Autodesk Inventor part; units mm, degrees
ref_plane "YZ Plane" through (0, 0, 0) normal (1, 0, 0) x (0, 1, 0)
ref_plane "XZ Plane" through (0, 0, 0) normal (0, 1, 0) x (-1, 0, 0)
ref_plane "XY Plane" through (0, 0, 0) normal (0, 0, 1) x (1, 0, 0)
sketch "Sketch1" plane through (0, 0, 0) normal (0, 0, 1) x (1, 0, 0)
  circle A0 centre (0, 0) radius 25
  circle A1 centre (0, 0) radius 23
  circle A2 centre (0, 0) radius 22
  circle A3 centre (0, 0) radius 20
  circle A4 centre (0, 0) radius 19
  circle A5 centre (0, 0) radius 17
  line L0 (25, 0) -> (-25, 0) construction
  line L1 (0, 25) -> (0, -25) construction
  dimension "d0" = 50
  dimension "d1" = 2
  dimension "d2" = 44
  dimension "d3" = 2
  dimension "d4" = 38
  dimension "d5" = 2
extrude "Extrusion2" add sketch "Sketch1" along normal blind 10 contours A0
sketch "Sketch2" plane through (0, 0, 0) normal (0, 1, 0) x (-1, 0, 0)
  line L0 (-23, 0) -> (23, 0) construction
  line L1 (23, 0) -> (-23, 0) construction
  line L2 (-23, 0) -> (-23, 10) construction
  line L3 (23, 10) -> (23, 0) construction
  line L4 (23, 10) -> (23, 0) construction
  circle A0 centre (23, 5) radius 2 construction
  line L5 (0, 0) -> (0, 10) construction
  circle A1 centre (-23, 5) radius 2 construction
  line L6 (24.0412, 3.2924) -> (23, 7)
  line L7 (-23, 0) -> (-23, 10)
  line L8 (23, 10) -> (23, 0) construction
  line L9 (-23, 5) -> (23, 5) construction
  line L10 (23, 10) -> (23, 0) construction
  circle A2 centre (-22.1677, 5) radius 2
  circle A3 centre (22.2113, 5) radius 2
  line L11 (20.2113, 5) -> (24.2113, 5)
  line L12 (-20.1677, 5) -> (-24.1677, 5)
  point P0 (-23, 7)
  point P1 (-23, 3)
  dimension "d12" = 4
  dimension "d11" = 10
  dimension "d31" = 46
  dimension "d32" = 4
  dimension "d33" = 4
revolve "Revolution1" add sketch "Sketch2" angle 360 about axis through (23, 0, 5) along (-1, 0, 0) picked at (21.3446, 5.1473) picked at (23.3511, 6.1311) contours L11 A3 L6 | L6 A3 L11
revolve "Revolution2" add sketch "Sketch2" angle 360 about axis through (23, 0, 5) along (-1, 0, 0) picked at (-23.13, 6.1339) picked at (-21.1282, 5.1469) contours L12 A2 L7 | L7 A2 L12
properties part number "probe_gimbal_prototype"
CAD build for the part. Positions are in the model's coordinates, mm. Coordinates: 2 decimals unless noted, no trailing zeros. Write each loop counter-clockwise with the first axis right and the second up, starting at its lowest first coordinate (ties: lowest second). Pieces come first, ordered by that corner, then holes. Notation, with made-up numbers: (7.25, 71.25) -> (28.25, 71.25) arc R11 ccw to (28.25, 84.25) -> close; hole circle Ø8 at (72.25, -35). An arc over 180 degrees is marked (long way). Return JSON: item names as keys, results as strings. Group by question number.
Q1. Cut at D-D, the plane y = 0. Give the cut face in (x, z), then the cut area to 3 significant figures.
Q2. Cut at C-C, the plane z = 2.25. Give the cut face in (x, y).
Q3. Pull direction Y, two halves, no side cores. Call faces 1 (the face through (23.846, -7.509, 4.93)), 2 (the face through (21.938, -6.909, 4.93)), 3 (the face through (22.1, -7.3, 0)): released by +Y, released by -Y, zero draft, split by the parting line, or undercut.
Q4. Flat gauge pins, fed straight in: pin 1 (6 mm diameter, centred on x = 3, z = 5.5, fed in from -Y); pin 2 (6 mm diameter, centred on x = 19.5, y = 17.5, fed in from +Z); pin 3 (2 mm diameter, centred on x = -1.5, z = 6, fed in from +Y) (3 decimals); pin 4 (3 mm diameter, centred on x = -8, z = 2, fed in from -Y). Where does each tip first touch, or does it go through?
Q5. Drill centre lines: line 1 (Y direction, x = 0, z = 5.25); line 2 (Y direction, x = -6, z = 3.75); line 3 (X direction, y = 11.5, z = 3). Where is each one in solid material? Low to high.
Q6. Cut at A-A, the plane x = 0. Give the cut face in (y, z).
Q7. Cut at B-B, the plane y = -20.5. Give the cut face in (x, z), then the cut area to 3 significant figures.
Returned:
{
 "1": {"outline": "(-25, 0) -> (-23, 0) -> (-23, 3.16) arc R2 ccw (long way) to (-23, 6.84) -> (-23, 10) -> (-25, 10) -> close; (23, 0) -> (25, 0) -> (25, 10) -> (23, 10) -> (23, 6.82) arc R2 ccw (long way) to (23, 3.18) -> close", "area": "58.9 mm2"},
 "2": {"outline": "circle Ø50 at (0, 0); hole circle Ø46 at (0, 0)"},
 "3": {"face 1": "split by the parting line", "face 2": "undercut", "face 3": "zero draft"},
 "4": {"pin 1": "stops at y = -25", "pin 2": "stops at z = 10", "pin 3": "stops at y = 24.995", "pin 4": "stops at y = -24.14"},
 "5": {"line 1": "y = -25 to -23, 23 to 25", "line 2": "y = -24.27 to -22.2, 22.2 to 24.27", "line 3": "x = -22.2 to -19.92, 19.92 to 22.2"},
 "6": {"outline": "(-25, 0) -> (-23, 0) -> (-23, 10) -> (-25, 10) -> close; (23, 0) -> (25, 0) -> (25, 10) -> (23, 10) -> close"},
 "7": {"outline": "(-14.31, 0) -> (-10.43, 0) -> (-10.43, 10) -> (-14.31, 10) -> close; (10.43, 0) -> (14.31, 0) -> (14.31, 10) -> (10.43, 10) -> close", "area": "77.6 mm2"}
}
